Model file for the job. Use its own axes, mm. A direction names the side the tool comes from. Coordinates: 2 decimals unless noted, no trailing zeros. Loops run counter-clockwise (first coordinate to the right, second up) from the corner with the lowest first, then second, coordinate; pieces in that order, holes last. Notation, with made-up numbers: (35, 18.25) - (42, 18.25) arc R11 cw to (42, 35.25) - close; hole circle Ø8 at (-36.75, 33). An arc over 180 degrees is marked (long way). Write each question's results on one line, items separated by ' | '. Start each with the question number.
```python
from build123d import *

# Parameters (mm, degrees)
SKETCH1_W                       = 9.13
SKETCH1_H                       = 0.3
BOSS_EXTRUDE1_DEPTH             = 11.42
BOSS_EXTRUDE2_DEPTH             = 2.535
FILLET1_R                       = 1.3
BOSS_EXTRUDE3_DEPTH             = 0.3
BOSS_EXTRUDE4_DEPTH             = 0.3
FILLET2_R                       = 0.3
FILLET3_R                       = 0.6
BOSS_EXTRUDE5_REACH             = 17.194
BOSS_EXTRUDE5_DIRECTION_2_REACH = 17.194
FILLET4_R                       = 0.595


with BuildPart() as part:
    # Sketch1 → Boss-Extrude1 (new body)
    with BuildSketch(Plane(origin=(0, 0, 0), x_dir=(1, 0, 0), z_dir=(0, 1, 0))):
        Rectangle(SKETCH1_W, SKETCH1_H)
    extrude(amount=BOSS_EXTRUDE1_DEPTH)

    # Sketch2 → Boss-Extrude2 (add, symmetric)
    with BuildSketch(Plane(origin=(0, 0, 0), x_dir=(0, 0, -1), z_dir=(1, 0, 0))):
        with BuildLine():
            Line((-0.15, 11.42), (0.15, 11.42))
            ThreePointArc((0.15, 11.42), (0.83370873, 12.245332078), (1.771840569, 11.727124282))
            Line((1.771840569, 11.727124282), (3.806143873, 6.548436218))
            ThreePointArc((3.806143873, 6.548436218), (3.904386052, 6.129654649), (3.879736877, 5.700210886))
            Line((3.879736877, 5.700210886), (3.610438676, 4.379957823))
            Line((3.610438676, 4.379957823), (3.904386052, 4.32))
            Line((3.904386052, 4.32), (4.173684252, 5.640253063))
            ThreePointArc((4.173684252, 5.640253063), (4.203263262, 6.155585579), (4.085372648, 6.658123461))
            Line((4.085372648, 6.658123461), (2.051069344, 11.836811525))
            ThreePointArc((2.051069344, 11.836811525), (0.77789042, 12.540093534), (-0.15, 11.42))
        make_face()
    extrude(amount=BOSS_EXTRUDE2_DEPTH, both=True)

    # Fillet1
    fillet1_edges = [part.edges().sort_by_distance(p)[0] for p in [
        (-2.535, 4.349978911, -3.757412364),
        (2.535, 4.349978911, -3.757412364),
    ]]
    fillet(fillet1_edges, radius=FILLET1_R)

    # Sketch3 → Boss-Extrude3 (add)
    with BuildSketch(Plane(origin=(0, 0, -0.15), x_dir=(-1, 0, 0), z_dir=(0, 0, -1))):
        with BuildLine():
            Line((-0.57, 0), (0.57, 0))
            Line((0.57, 0), (0.57, -1.6))
            Line((0.57, -1.6), (0.33, -2.770784784))
            ThreePointArc((0.33, -2.770784784), (0, -3.04), (-0.33, -2.770784784))
            Line((-0.33, -2.770784784), (-0.57, -1.6))
            Line((-0.57, -1.6), (-0.57, 0))
        make_face()
    extrude(amount=-BOSS_EXTRUDE3_DEPTH)

    # Sketch4 → Boss-Extrude4 (add)
    with BuildSketch(Plane(origin=(4.565, 0, 0), x_dir=(0, 0, -1), z_dir=(1, 0, 0))):
        with BuildLine():
            Line((-0.15, 11.42), (-0.15, 0))
            Line((-0.15, 0), (-1.425, 0))
            Line((-1.425, 0), (-1.425, 0.4))
            ThreePointArc((-1.425, 0.4), (-1.925, 0.9), (-2.425, 0.4))
            Line((-2.425, 0.4), (-2.425, 0))
            Line((-2.425, 0), (-3.615, 0))
            Line((-3.615, 0), (-3.615, 0.4))
            ThreePointArc((-3.615, 0.4), (-4.115, 0.9), (-4.615, 0.4))
            Line((-4.615, 0.4), (-4.615, 0))
            Line((-4.615, 0), (-6.19, 0))
            Line((-6.19, 0), (-6.19, 0.9))
            Line((-6.19, 0.9), (-2.4, 10.767226789))
            ThreePointArc((-2.4, 10.767226789), (-2.026327352, 11.241078061), (-1.45, 11.42))
            Line((-1.45, 11.42), (-0.15, 11.42))
        make_face()
    boss_extrude4 = extrude(amount=-BOSS_EXTRUDE4_DEPTH)

    # Fillet2
    fillet2_edges = [part.edges().sort_by_distance(p)[0] for p in [
        (4.265, 5.71, 0.15),
    ]]
    fillet(fillet2_edges, radius=FILLET2_R)

    # Fillet3
    fillet3_edges = [part.edges().sort_by_distance(p)[0] for p in [
        (4.565, 5.71, -0.15),
    ]]
    fillet(fillet3_edges, radius=FILLET3_R)

    # Boss-Extrude5: up to this face of the body (flat: up to its plane)
    boss_extrude5_end = Plane(part.part.faces().sort_by_distance((4.415, 0.2, 2.425))[0])
    # Sketch5 → Boss-Extrude5 (add, up to the picked face)
    with BuildSketch(Plane(origin=(0, 0, 3.02), x_dir=(-1, 0, 0), z_dir=(0, 0, -1)), mode=Mode.PRIVATE) as boss_extrude5_sk1:
        with BuildLine():
            Line((-4.565, 0), (-4.265, 0))
            Line((-4.265, 0), (-4.265, -0.734365081))
            ThreePointArc((-4.265, -0.734365081), (-4.31067228, -0.963975141), (-4.440735931, -1.15862915))
            Line((-4.440735931, -1.15862915), (-4.833553391, -1.551446609))
            ThreePointArc((-4.833553391, -1.551446609), (-4.966005966, -1.787534255), (-4.95599841, -2.058053958))
            Line((-4.95599841, -2.058053958), (-4.422200477, -3.718167625))
            Line((-4.422200477, -3.718167625), (-4.707799523, -3.81))
            Line((-4.707799523, -3.81), (-5.241597456, -2.149886332))
            ThreePointArc((-5.241597456, -2.149886332), (-5.257609545, -1.717054807), (-5.045685425, -1.339314575))
            Line((-5.045685425, -1.339314575), (-4.652867966, -0.946497116))
            ThreePointArc((-4.652867966, -0.946497116), (-4.58783614, -0.849170111), (-4.565, -0.734365081))
            Line((-4.565, -0.734365081), (-4.565, 0))
        make_face()
    boss_extrude5_tool1 = split(extrude(boss_extrude5_sk1.sketch, amount=BOSS_EXTRUDE5_REACH, mode=Mode.PRIVATE), bisect_by=boss_extrude5_end, keep=Keep.BOTH, mode=Mode.PRIVATE)
    boss_extrude5 = boss_extrude5_tool1.solids().sort_by(Axis((4.415, -0.039429, 3.02), (0, 0, -1)))[0]
    add(boss_extrude5)

    # Boss-Extrude5 direction 2: up to this face of the body (flat: up to its plane)
    boss_extrude5_direction_2_end = Plane(part.part.faces().sort_by_distance((4.415, 0.2, 3.615))[0])
    # Sketch5 → Boss-Extrude5 direction 2 (add, up to the picked face)
    with BuildSketch(Plane(origin=(0, 0, 3.02), x_dir=(-1, 0, 0), z_dir=(0, 0, -1)), mode=Mode.PRIVATE) as boss_extrude5_direction_2_sk1:
        with BuildLine():
            Line((-4.565, 0), (-4.265, 0))
            Line((-4.265, 0), (-4.265, -0.734365081))
            ThreePointArc((-4.265, -0.734365081), (-4.31067228, -0.963975141), (-4.440735931, -1.15862915))
            Line((-4.440735931, -1.15862915), (-4.833553391, -1.551446609))
            ThreePointArc((-4.833553391, -1.551446609), (-4.966005966, -1.787534255), (-4.95599841, -2.058053958))
            Line((-4.95599841, -2.058053958), (-4.422200477, -3.718167625))
            Line((-4.422200477, -3.718167625), (-4.707799523, -3.81))
            Line((-4.707799523, -3.81), (-5.241597456, -2.149886332))
            ThreePointArc((-5.241597456, -2.149886332), (-5.257609545, -1.717054807), (-5.045685425, -1.339314575))
            Line((-5.045685425, -1.339314575), (-4.652867966, -0.946497116))
            ThreePointArc((-4.652867966, -0.946497116), (-4.58783614, -0.849170111), (-4.565, -0.734365081))
            Line((-4.565, -0.734365081), (-4.565, 0))
        make_face()
    boss_extrude5_direction_2_tool1 = split(extrude(boss_extrude5_direction_2_sk1.sketch, amount=-BOSS_EXTRUDE5_DIRECTION_2_REACH, mode=Mode.PRIVATE), bisect_by=boss_extrude5_direction_2_end, keep=Keep.BOTH, mode=Mode.PRIVATE)
    boss_extrude5_direction_2 = boss_extrude5_direction_2_tool1.solids().sort_by(Axis((4.415, -0.039429, 3.02), (0, 0, 1)))[0]
    add(boss_extrude5_direction_2)

    # Fillet4
    fillet4_edges = [part.edges().sort_by_distance(p)[0] for p in [
        (4.565, -3.764083813, 2.425),
        (4.565, -3.764083813, 3.615),
    ]]
    fillet(fillet4_edges, radius=FILLET4_R - 0.0001)  # a hair under: the kernel refuses the full size

    # Mirror1: Boss-Extrude4, Boss-Extrude5, Boss-Extrude5 direction 2 across plane
    add(boss_extrude4.mirror(Plane(origin=(0, 0, 0), x_dir=(0, 0, 1), z_dir=(1, 0, 0))))
    add(boss_extrude5.mirror(Plane(origin=(0, 0, 0), x_dir=(0, 0, 1), z_dir=(1, 0, 0))))
    add(boss_extrude5_direction_2.mirror(Plane(origin=(0, 0, 0), x_dir=(0, 0, 1), z_dir=(1, 0, 0))))


solid = part.part
```
Q1. Which spindle directions (+Z, -Z, +X, -X, +Y, -Y) get a long thin tool onto all of the face, cutting with end or side? Do faces 1 (the flat face through (0.035, 5.049, -3.747)), 2 (the flat face through (0, 6, -0.15)), 3 (the flat face through (4.565, 5, 3)), 4 (the flat face through (-4.69, -2.88, 3.01)). Say none if no direction does.
Q2. Cut at A-A (y = 9.5). List the corners of the cut face in (x, z) (3 decimals).
Q3. Drill centre lines: L1, parallel to X at y = 5, z = 0.75 (3 decimals); L2, parallel to Z at x = -2, y = 2. Where is each one in solid material? Low to high. Write a range as from..to.
Q4. Cut at D-D (y = 4). List the corners of the cut face in (x, z) (3 decimals), and give its area (3 significant figures).
Q5. Mould opens along Z. For faces 5 (the cylindrical face through (0.035, 6.136, -3.904)), 6 (the cylindrical face through (0.035, 6.148, -4.204)), 7 (the cylindrical face through (-5.26, -1.72, 3.01)), 8 (the cylindrical face through (0.035, 12.544, -0.8)) say: +Z half, -Z half, draft (parallel to the pull), parting line (faces both ways), or undercut.
Q6. Cut at B-B (z = 5.5). List the corners of the cut face in (x, y) (3 decimals).
Q7. Pin check, flat tips, straight feed: pin 1 (1.5 mm diameter, centred on x = -1.5, y = 3, fed in from +Z); pin 2 (1.7 mm diameter, centred on x = 3, z = 0.5, fed in from -Y); pin 3 (3 mm diameter, centred on y = 0, z = 2, fed in from -X). Stop position of each tip, or through.
Q8. Cut at C-C (x = -1). List the corners of the cut face in (y, z).
Check result:
1) face 1: +X, -X | face 2: +X, -X, -Y | face 3: +Z, -Z, +X, +Y | face 4: +Z, -Z
2) outline: (-4.565, -0.15) - (3.965, -0.15) arc R0.6 ccw to (4.565, 0.45) - (4.565, 2.887) - (4.265, 2.887) - (4.265, 0.45) arc R0.3 cw to (3.965, 0.15) - (-4.265, 0.15) - (-4.265, 2.887) - (-4.565, 2.887) - close; (-2.535, -2.969) - (2.535, -2.969) - (2.535, -2.647) - (-2.535, -2.647) - close
3) L1: -4.565..-4.265, 4.265..4.565 | L2: -0.15..0.15
4) outline: (-4.565, -0.15) - (3.965, -0.15) arc R0.6 ccw to (4.565, 0.45) - (4.565, 4.999) - (4.265, 4.999) - (4.265, 0.45) arc R0.3 cw to (3.965, 0.15) - (-4.265, 0.15) - (-4.265, 4.999) - (-4.565, 4.999) - close | area: 5.59 mm²
5) face 5: undercut | face 6: -Z half | face 7: draft | face 8: parting line
6) outline: (-4.565, 0) - (-4.265, 0) - (-4.265, 2.696) - (-4.565, 2.696) - close; (4.265, 0) - (4.565, 0) - (4.565, 2.696) - (4.265, 2.696) - close
7) pin 1: z = 0.15 | pin 2: y = 0 | pin 3: x = -5.13
8) outline: (0, -0.15) - (11.42, -0.15) arc R0.84 cw to (11.73, -1.77) - (6.55, -3.81) arc R1.5 cw to (5.7, -3.88) - (4.38, -3.61) - (4.32, -3.9) - (5.64, -4.17) arc R1.8 ccw to (6.66, -4.09) - (11.84, -2.05) arc R1.14 ccw to (11.42, 0.15) - (0, 0.15) - close
